Design review of the part built by this model. Coordinates are the model's own, in mm. Face numbers are marked on the shaded views. A direction names the side the tool comes from. Coordinates: 2 decimals unless noted, no trailing zeros. Write each loop counter-clockwise with the first axis right and the second up, starting at its lowest first coordinate (ties: lowest second). Pieces come first, ordered by that corner, then holes. Notation, with made-up numbers: (61, 20.25) - (99, 20.25) arc R21 cw to (99, 38.25) - close; hole circle Ø9 at (12.25, 68). An arc over 180 degrees is marked (long way). Answer as a JSON object with one key per item and string values.
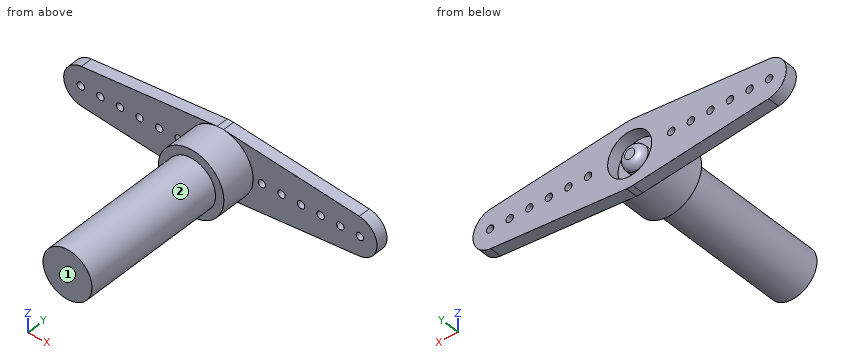
Autodesk Inventor part; units mm, degrees
ref_plane "YZ Plane" through (0, 0, 0) normal (1, 0, 0) x (0, 1, 0)
ref_plane "XZ Plane" through (0, 0, 0) normal (0, 1, 0) x (-1, 0, 0)
ref_plane "XY Plane" through (0, 0, 0) normal (0, 0, 1) x (1, 0, 0)
sketch "Sketch1" plane through (0, 0, 0) normal (0, 1, 0) x (-1, 0, 0)
  circle A0 centre (0, 0) radius 2.5
  dimension "d0" = 5
extrude "Extrusion1" add sketch "Sketch1" along normal blind 9.5 and the other way blind 10
sketch "Sketch2" plane through (0, 9.5, 0) normal (0, 1, 0) x (1, 0, 0)
  line L0 (0, 0) -> (-16, 0) construction
  line L1 (0, 0) -> (0, 3.35) construction
  arc A0 (-14.1929, 1.9907) -> (-14.1929, -1.9907) centre (-14, 0) ccw
  line L2 (-14.1929, -1.9907) -> (-0.323, -3.3344)
  line L3 (-14.1929, 1.9907) -> (-0.323, 3.3344)
  arc A1 (14.1929, -1.9907) -> (14.1929, 1.9907) centre (14, 0) ccw
  line L4 (14.1929, -1.9907) -> (0.323, -3.3344)
  line L5 (14.1929, 1.9907) -> (0.323, 3.3344)
  circle A2 centre (0, 0) radius 2.5
  arc A3 (-0.323, -3.3344) -> (0.323, -3.3344) centre (0, 0) ccw
  arc A4 (0.323, 3.3344) -> (-0.323, 3.3344) centre (0, 0) ccw
  dimension "d5" = 16
  dimension "d7" = 4
  dimension "d8" = 2
  dimension "d11" = 0.85
extrude "Extrusion2" add sketch "Sketch2" against normal blind 1.2
sketch "Sketch3" plane through (0, 8.3, 0) normal (0, -1, 0) x (1, 0, 0)
  circle A0 centre (0, 0) radius 2.5
  circle A1 centre (0, 0) radius 3.35
extrude "Extrusion3" add sketch "Sketch3" along normal blind 3.5
sketch "Sketch4" plane through (0, 9.5, 0) normal (0, 1, 0) x (1, 0, 0)
  circle A0 centre (0, 0) radius 2.25
  dimension "d16" = 4.5
extrude "Extrusion4" cut sketch "Sketch4" against normal blind 1.25
sketch "Sketch5" plane through (0, 8.25, 0) normal (0, 1, 0) x (1, 0, 0)
  circle A0 centre (0, 0) radius 1.25
  dimension "d19" = 2.5
extrude "Extrusion5" add sketch "Sketch5" along normal blind 1.25
fillet "Fillet1" radius 0.74 1 edges at (-1.25, 9.5, 0)
sketch "Sketch6" plane through (0, 9.5, 0) normal (0, 1, 0) x (1, 0, 0)
  circle A0 centre (-4.25, 0) radius 0.375
  line L0 (0, 0) -> (-16, 0) construction
  arc A1 (-14.1929, 1.9907) -> (-14.1929, -1.9907) centre (-14, 0) ccw construction
  circle A2 centre (-6.25, 0) radius 0.375
  circle A3 centre (-8.25, 0) radius 0.375
  circle A4 centre (-10.25, 0) radius 0.375
  circle A5 centre (-12.25, 0) radius 0.375
  circle A6 centre (-14.25, 0) radius 0.375
  dimension "d23" = 0.75
  dimension "d24" = 4.25
  dimension "d27" = 2
extrude "Extrusion6" cut sketch "Sketch6" against normal blind 2.8375
mirror "Mirror1" about plane through (0, 0, 0) normal (1, 0, 0) of "Extrusion6"
properties part number "Servo shaft and horn"
(1) Take a section at A-A, the plane x = 12.25. Write out the cut boundary in (y, z) (3 decimals).
Solved:
{"outline": "(8.3, -2.179) - (9.5, -2.179) - (9.5, -0.375) - (8.3, -0.375) - close; (8.3, 0.375) - (9.5, 0.375) - (9.5, 2.179) - (8.3, 2.179) - close"}
(2) To check wall thickness, follow line 1 (Z direction, x = -14.25, y = 8.7) (3 decimals); line 2 (Y direction, x = -2, z = -2); line 3 (Y direction, x = -6, z = -1). State the ranges of each line that lie inside material, in increasing order. Write a range as from..to.
Solved:
{"line 1": "z = -1.984..-0.375, 0.375..1.984", "line 2": "y = 4.8..9.5", "line 3": "y = 8.3..9.5"}
(3) For pin 1 (1 mm diameter, centred on y = -5, z = 2, fed in from +X); pin 2 (3 mm diameter, centred on x = -4.5, z = 0.5, fed in from -Y); pin 3 (1.5 mm diameter, centred on y = -4.5, z = -1.5, fed in from -X), all flat-tipped, find the tip position at first contact; note any pin that passes through.
Solved:
{"pin 1": "stops at x = 2", "pin 2": "stops at y = 4.8", "pin 3": "stops at x = -2.38"}
(4) Take a section at C-C, the plane y = 2.75. Write out the cut boundary in (x, z).
Solved:
{"outline": "circle Ø5 at (0, 0)"}
(5) Take a section at B-B, the plane x = 6.25. Write out the cut boundary in (y, z) (3 decimals).
Solved:
{"outline": "(8.3, -2.76) - (9.5, -2.76) - (9.5, -0.375) - (8.3, -0.375) - close; (8.3, 0.375) - (9.5, 0.375) - (9.5, 2.76) - (8.3, 2.76) - close"}
(6) Tool access review of the marked faces 1 and 2: name each direction out of +Z, -Z, +X, -X, +Y, -Y from which nothing blocks a thin tool from reaching the whole face with its end or side.
Solved:
{"face 1": "+Z, -Z, +X, -X, -Y", "face 2": "-Y"}
